Could you check a few things on this model? Use its own coordinates, in mm. Coordinates: 2 decimals unless noted, no trailing zeros. Order: outer loops, then holes, each group sorted by start corner. A loop starts at its lowest first (then second) coordinate and runs counter-clockwise, first axis right, second up.
```python
from build123d import *

# Parameters (mm, degrees)
SKETCH1_W          = 8
SKETCH1_H          = 1
CHAMFER1_SIZE      = 0.3
CUT_EXTRUDE2_DEPTH = 0.84


with BuildPart() as part:
    # Sketch1 → Revolve1 (revolve)
    with BuildSketch(Plane(origin=(0, 0, 0), x_dir=(0, 0, -1), z_dir=(1, 0, 0))):
        with Locations((4, 0.5)):
            Rectangle(SKETCH1_W, SKETCH1_H)
    revolve(axis=Axis((0, 0, -8), (0, 0, 1)))

    # Chamfer1
    chamfer1_edges = [part.edges().sort_by_distance(p)[0] for p in [
        (0, -1, -8),
    ]]
    chamfer(chamfer1_edges, length=CHAMFER1_SIZE)

    # Sketch7 → Revolve2 (revolve)
    with BuildSketch(Plane(origin=(0, 0, 0), x_dir=(0, 0, -1), z_dir=(1, 0, 0)), mode=Mode.PRIVATE) as revolve2_sk:
        Polygon((0, 2), (0.2, 2), (1.2, 1), (1.2, 0), (0, 0), align=None)
    revolve(revolve2_sk.sketch.rotate(Axis((0, 0, 0), (0, 0, -1)), 180), axis=Axis((0, 0, 0), (0, 0, -1)))

    # Boss-Extrude1 cone 1 section (through the dimple's axis) → Boss-Extrude1 (revolve)
    with BuildSketch(Plane(origin=(0, 0, -1.2), x_dir=(0, -1, 0), z_dir=(1, 0, 0))):
        Polygon((0, 0), (1, 0), (0, 1), align=None)
    revolve(axis=Axis((0, 0, -1.2), (0, 0, -1)))

    # Sketch5 → Cut-Extrude2 (cut)
    with BuildSketch(Plane.XY):
        Polygon((0.65, -0.375277675), (0.65, 0.375277675), (0, 0.75055535), (-0.65, 0.375277675), (-0.65, -0.375277675), (0, -0.75055535), align=None)
    extrude(amount=-CUT_EXTRUDE2_DEPTH, mode=Mode.SUBTRACT)

    # Cut-Extrude3 cone 1 section (through the dimple's axis) → Cut-Extrude3 (revolve, cut)
    with BuildSketch(Plane(origin=(0, 0, 0), x_dir=(0, -1, 0), z_dir=(1, 0, 0))):
        Polygon((0, 0), (0.75055535, 0), (0, 0.75055535), align=None)
    revolve(axis=Axis((0, 0, 0), (0, 0, -1)), mode=Mode.SUBTRACT)


solid = part.part
```
Item 1: Suppose I cut it at B-B (z = -5.5). List the corners of the cut face in (x, y) for me.
Item 2: Suppose I cut it at A-A (y = 0). List the corners of the cut face in (x, z) for me, and give its area (3 significant figures).
Item 3: I need wall thicknesses on line 1 (Z direction, x = 0.1, y = -0.25); line 2 (Z direction, x = 0.85, y = -0.85); line 3 (Y direction, x = 0.5, z = -7.25). Which ranges of each line are inside material? Lowest first, please.
Item 4: Thinking about a two-plate mould opening in Y: for faces 1 (the face through (1, 0, -4)), 2 (the face through (0, 0, -0.84)), 3 (the face through (0, 1, 0)), which applies, +Y half, -Y half, draft (parallel to the pull), parting line (faces both ways), or undercut?
Item 5: For pin 1 Ø1 at (y, z) = (-1, -4) entering from +X; pin 2 Ø1 at (y, z) = (0.5, -3) entering from -X; pin 3 Ø2 at (x, z) = (0, -3) entering from -Y, each with a flat end and sliding along its axis, tell me the tip position at first contact or that it passes through.
Geometry results:
1. outline: circle Ø2 at (0, 0)
2. outline: (-2, -0.2) - (-1, -1.2) - (-1, -7.7) - (-0.7, -8) - (0.7, -8) - (1, -7.7) - (1, -1.2) - (2, -0.2) - (2, 0) - (0.75, 0) - (0.65, -0.1) - (0.65, -0.84) - (-0.65, -0.84) - (-0.65, -0.1) - (-0.75, 0) - (-2, 0) - close
2. area: 16.2 mm2
3. line 1: z = -8 to -0.84
3. line 2: z = -1 to 0
3. line 3: y = -0.87 to 0.87
4. face 1: parting line
4. face 2: undercut
4. face 3: draft
5. pin 1: stops at x = 0.87
5. pin 2: stops at x = -1
5. pin 3: stops at y = -1
